Job drawing, mm, ordinate dimensions from the low corner. One solid piece. A direction names the side the tool comes from. Coordinates: 2 decimals unless noted, no trailing zeros. Write each loop counter-clockwise with the first axis right and the second up, starting at its lowest first coordinate (ties: lowest second). Pieces come first, ordered by that corner, then holes. Notation, with made-up numbers: (9.5, 47.25) - (40.5, 47.25) arc R12 cw to (40.5, 64.25) - close; hole circle Ø10 at (71.5, 37). An arc over 180 degrees is marked (long way). Use one line per item in the form item = value. Start each with the question number.
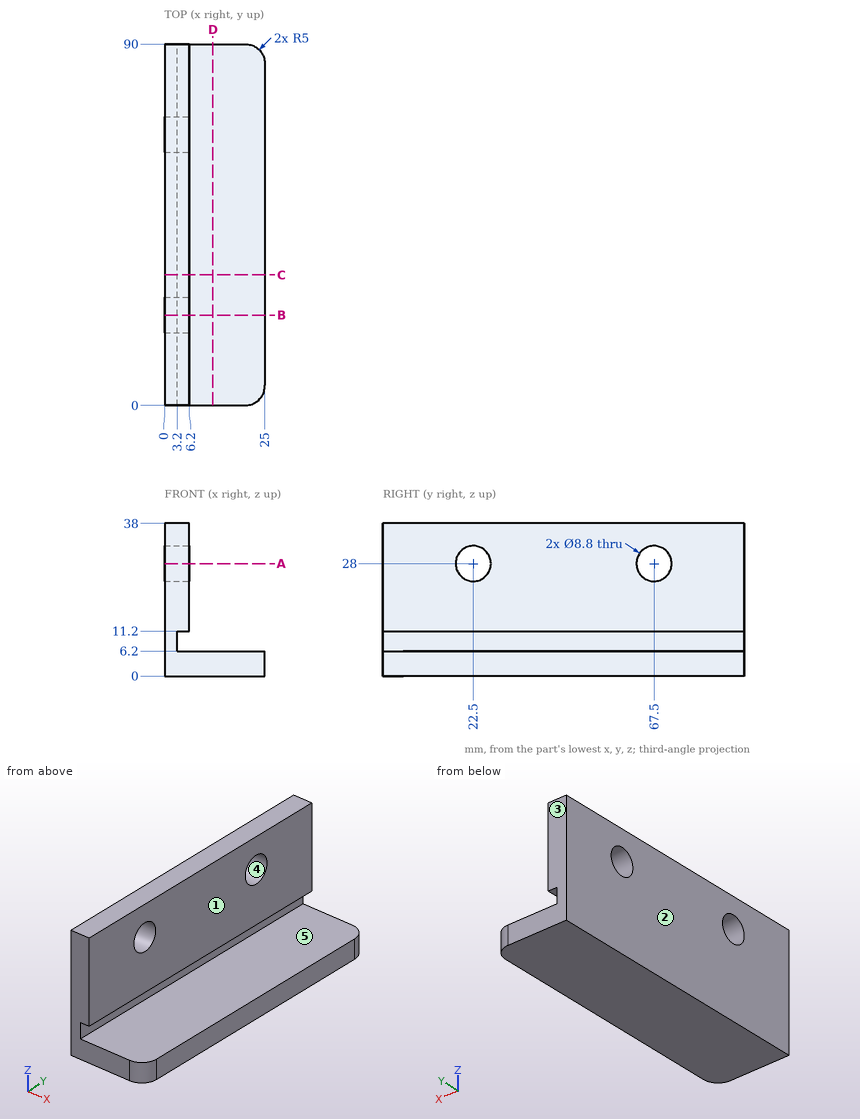
Q1. Mould opens along Y. For the marked faces 3, 4 and 5 say: released by +Y, released by -Y, zero draft, split by the parting line, or undercut.
Q2. Slice it at C-C (y = 32.5). List the corners of the cut face in (x, z).
Q3. Pin check, flat tips, straight feed: P1, Ø3, axis at y = 12, z = 20.5, coming from the +X side; P2, Ø1.5, axis at x = 8.5, y = 60.5, coming from the +Z side. Stop position of each tip, or through.
Q4. Which spindle directions (+Z, -Z, +X, -X, +Y, -Y) get a long thin tool onto all of the face, cutting with end or side? Do the marked faces 1 and 2. Say none if no direction does.
Q5. Slice it at B-B (y = 22.5). List the corners of the cut face in (x, z), plus the area to 3 significant figures.
Q6. Slice it at A-A (z = 28). List the corners of the cut face in (x, y).
Q7. Drill centre lines: probe 1 along Z at (x, y) = (5.25, 22.5); probe 2 along Z at (x, y) = (1.5, 22.5); probe 3 along X at (y, z) = (32, 17.5). Where is each one in solid material? Low to high.
Q8. Slice it at D-D (x = 12). List the corners of the cut face in (y, z).
Solution:
q1.face_3 = released by +Y
q1.face_4 = undercut
q1.face_5 = zero draft
q2.outline = (0, 0) - (25, 0) - (25, 6.2) - (3.2, 6.2) - (3.2, 11.2) - (6.2, 11.2) - (6.2, 38) - (0, 38) - close
q3.P1 = 6.2
q3.P2 = 6.2
q4.face_1 = +Z, +X, +Y, -Y
q4.face_2 = +Z, -Z, -X, +Y, -Y
q5.outline = (0, 0) - (25, 0) - (25, 6.2) - (3.2, 6.2) - (3.2, 11.2) - (6.2, 11.2) - (6.2, 23.6) - (0, 23.6) - close; (0, 32.4) - (6.2, 32.4) - (6.2, 38) - (0, 38) - close
q5.area = 283 mm2
q6.outline = (0, 0) - (6.2, 0) - (6.2, 18.1) - (0, 18.1) - close; (0, 26.9) - (6.2, 26.9) - (6.2, 63.1) - (0, 63.1) - close; (0, 71.9) - (6.2, 71.9) - (6.2, 90) - (0, 90) - close
q7.probe_1 = 0 to 6.2, 11.2 to 23.6, 32.4 to 38
q7.probe_2 = 0 to 23.6, 32.4 to 38
q7.probe_3 = 0 to 6.2
q8.outline = (0, 0) - (90, 0) - (90, 6.2) - (0, 6.2) - close
